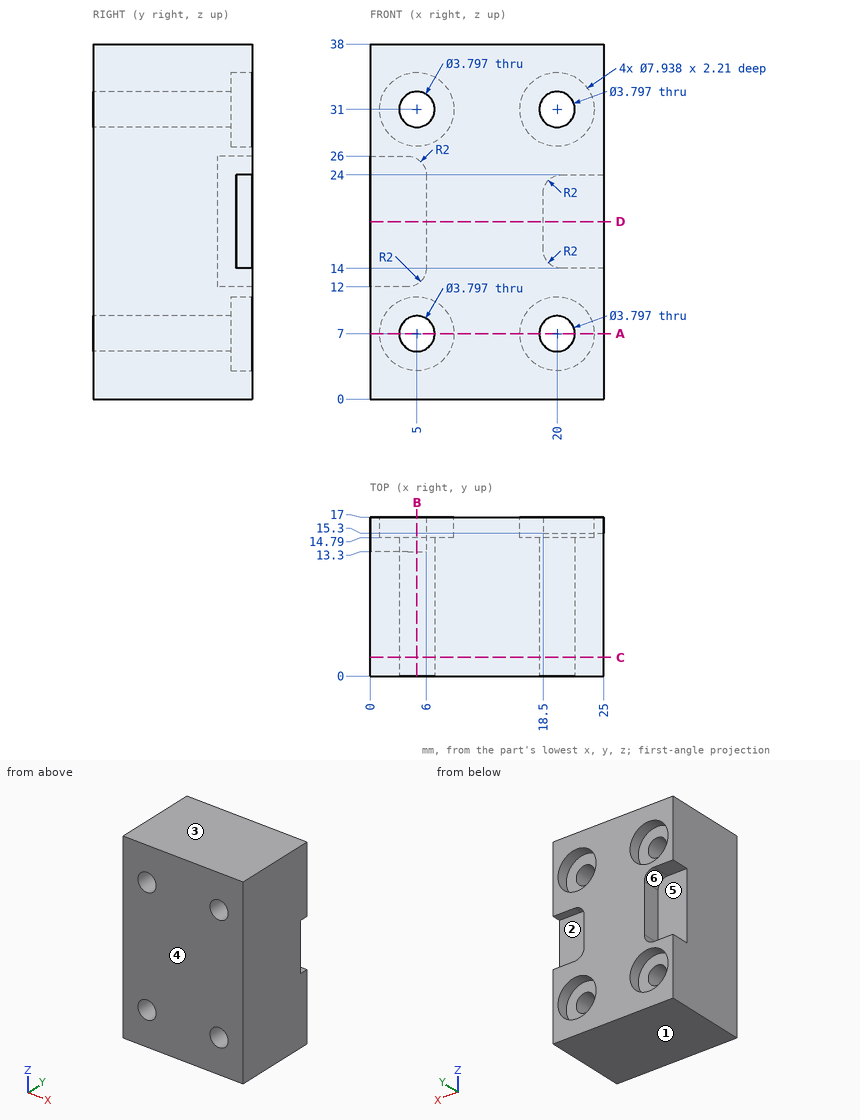
Design review of the part shown in the three views and the two pictorial views. Dimensions are in mm from the part's minimum x, y and z. A direction names the side the tool comes from. Give positions to 0.01 mm unless a question says otherwise; leave off trailing zeros. Loops run counter-clockwise (first coordinate to the right, second up) from the corner with the lowest first, then second, coordinate; pieces in that order, holes last. Notation, with made-up numbers: (72, -9.75) -> (122, -9.75) arc R27 ccw to (122, 11.25) -> close; hole circle Ø1 at (30.25, -34). An arc over 180 degrees is marked (long way). Write each question's results on one line, items separated by ' | '.
Q1. Take a section at D-D, the plane z = 19. Write out the cut boundary in (x, y), plus the area to 3 significant figures.
Reply:
outline: (0, 0) -> (25, 0) -> (25, 15.3) -> (18.5, 15.3) -> (18.5, 17) -> (6, 17) -> (6, 13.3) -> (0, 13.3) -> close | area: 392 mm²
Q2. Wall thickness on L1, parallel to X at y = 15.55, z = 31; L2, parallel to X at y = 9, z = 7; L3, parallel to Z at x = 20, y = 7.75: over which ranges is each line inside the solid? List them lowest first.
Reply:
L1: x = 0 to 1.03, 8.97 to 16.03, 23.97 to 25 | L2: x = 0 to 3.1, 6.9 to 18.1, 21.9 to 25 | L3: z = 0 to 5.1, 8.9 to 29.1, 32.9 to 38
Q3. Take a section at B-B, the plane x = 5. Write out the cut boundary in (y, z), plus the area to 3 significant figures.
Reply:
outline: (0, 0) -> (17, 0) -> (17, 3.03) -> (14.79, 3.03) -> (14.79, 5.1) -> (0, 5.1) -> close; (0, 8.9) -> (14.79, 8.9) -> (14.79, 10.97) -> (17, 10.97) -> (17, 12.27) -> (13.3, 12.27) -> (13.3, 25.73) -> (17, 25.73) -> (17, 27.03) -> (14.79, 27.03) -> (14.79, 29.1) -> (0, 29.1) -> close; (0, 32.9) -> (14.79, 32.9) -> (14.79, 34.97) -> (17, 34.97) -> (17, 38) -> (0, 38) -> close | area: 449 mm²
Q4. Machinability: for the marked faces 1 and 2, which of the approach directions +Z, -Z, +X, -X, +Y, -Y give a long, thin tool a straight path to every point of the face, cutting with its end or side? Answer none if there is none.
Reply:
face 1: -Z, +X, -X, +Y, -Y | face 2: +X, +Y
Q5. Take a section at A-A, the plane z = 7. Write out the cut boundary in (x, y).
Reply:
outline: (0, 0) -> (3.1, 0) -> (3.1, 14.79) -> (1.03, 14.79) -> (1.03, 17) -> (0, 17) -> close; (6.9, 0) -> (18.1, 0) -> (18.1, 14.79) -> (16.03, 14.79) -> (16.03, 17) -> (8.97, 17) -> (8.97, 14.79) -> (6.9, 14.79) -> close; (21.9, 0) -> (25, 0) -> (25, 17) -> (23.97, 17) -> (23.97, 14.79) -> (21.9, 14.79) -> close
Q6. The part is to be moulded in two halves that separate along Z. For the marked faces 3, 4, 5 and 6, say which applies: +Z half, -Z half, draft (parallel to the pull), parting line (faces both ways), or undercut.
Reply:
face 3: +Z half | face 4: draft | face 5: undercut | face 6: undercut
Q7. For pin 1 Ø5 at (x, z) = (23, 17) entering from +Y; pin 2 Ø1.4 at (y, z) = (16.5, 19) entering from +X; pin 3 Ø2.5 at (x, z) = (21.5, 5) entering from +Y, all flat-tipped, find the tip position at first contact; note any pin that passes through.
Reply:
pin 1: stops at y = 15.3 | pin 2: stops at x = 18.5 | pin 3: stops at y = 14.79
Q8. Take a section at C-C, the plane y = 2. Write out the cut boundary in (x, z).
Reply:
outline: (0, 0) -> (25, 0) -> (25, 38) -> (0, 38) -> close; hole circle Ø3.8 at (5, 7); hole circle Ø3.8 at (5, 31); hole circle Ø3.8 at (20, 7); hole circle Ø3.8 at (20, 31)
